Autodesk Inventor part; units mm, degrees
ref_plane "YZ Plane" through (0, 0, 0) normal (1, 0, 0) x (0, 1, 0)
ref_plane "XZ Plane" through (0, 0, 0) normal (0, 1, 0) x (-1, 0, 0)
ref_plane "XY Plane" through (0, 0, 0) normal (0, 0, 1) x (1, 0, 0)
sketch "Sketch2" plane through (0, 0, 0) normal (0, 1, 0) x (-1, 0, 0)
  circle A0 centre (0, 0) radius 22
  circle A1 centre (0, 0) radius 30
  dimension "d0" = 44
  dimension "d1" = 60
extrude "Extrusion1" add sketch "Sketch2" along normal blind 10
sketch "Sketch3" plane through (0, 10, 0) normal (0, 1, 0) x (1, 0, 0)
  circle A0 centre (0, 0) radius 30
  circle A1 centre (0, 0) radius 15
  dimension "d4" = 30
extrude "Extrusion2" add sketch "Sketch3" along normal blind 10
sketch "Sketch4" plane through (0, 20, 0) normal (0, 1, 0) x (1, 0, 0)
  circle A0 centre (0, 0) radius 25.1
  circle A1 centre (0, 0) radius 30
  dimension "d7" = 60
  dimension "d8" = 50.2
extrude "Extrusion3" add sketch "Sketch4" along normal blind 5
properties part number "smallbearingcup" material "Steel"
Here's how the part is built. I have some questions about the finished solid (model axes, mm). A direction names the side the tool comes from. Round coordinates to 2 decimals unless told otherwise and drop trailing zeros. Order: outer loops, then holes, each group sorted by start corner. A loop starts at its lowest first (then second) coordinate and runs counter-clockwise, first axis right, second up. Notation, with made-up numbers: M 39.25,76 L 59.25,76 A21 cw 59.25,113 Z; hole C 40,42.25 d6. An arc over 180 degrees is marked long. One line per question, with ' | ' between items.
1) I need wall thicknesses on line 1 (X direction, y = 17.25, z = 0); line 2 (X direction, y = 7.5, z = -0.5); line 3 (Z direction, x = 0, y = 22.65). Which ranges of each line are inside material? Lowest first, please.
Checked values:
line 1: x = -30 to -15, 15 to 30 | line 2: x = -30 to -21.99, 21.99 to 30 | line 3: z = -30 to -25.1, 25.1 to 30
2) Imagine slicing it at D-D, the plane y = 20.75. Write out the boundary of the cut face in (x, z).
Checked values:
outline: C 0,0 d60; hole C 0,0 d50.2
3) Imagine slicing it at B-B, the plane y = 11.5. Write out the boundary of the cut face in (x, z).
Checked values:
outline: C 0,0 d60; hole C 0,0 d30
4) On a 3-axis mill with a long thin cutter (end or side, diameter ignored), from which of +Z, -Z, +X, -X, +Y, -Y can I reach the whole of each face in a straight line? I mean faces 1 (the flat face through (14.4, 10, -5.2)), 2 (the flat face through (11, 20, 11)), 3 (the flat face through (-18, 25, 18)). Say none if no direction works.
Checked values:
face 1: -Y | face 2: +Y | face 3: +Z, -Z, +X, -X, +Y
5) I'm going to push flat-ended pins straight in: pin 1 Ø5 at (y, z) = (18.5, 16) entering from -X; pin 2 Ø1 at (y, z) = (18, -3) entering from -X; pin 3 Ø8 at (x, y) = (-9.5, 6.5) entering from +Z; pin 4 Ø25 at (x, z) = (-1, 0) entering from +Y. Where does each tip first touch, or does it pass through?
Checked values:
pin 1: stops at x = -26.79 | pin 2: stops at x = -29.9 | pin 3: stops at z = 29.49 | pin 4: passes through
6) We'd pull the mould along X, two halves only. Please class faces 4 (the flat face through (16, 0, 16)), 5 (the cylindrical face through (23.186, 22.465, -9.613)): released by +X, released by -X, zero draft, split by the parting line, or undercut.
Checked values:
face 4: zero draft | face 5: undercut
7) Imagine slicing it at A-A, the plane z = -12. Write out the boundary of the cut face in (x, y), plus the area to 3 significant figures.
Checked values:
outline: M -27.5,0 L -18.44,0 L -18.44,10 L -9,10 L -9,20 L -22.05,20 L -22.05,25 L -27.5,25 Z; M 9,10 L 18.44,10 L 18.44,0 L 27.5,0 L 27.5,25 L 22.05,25 L 22.05,20 L 9,20 Z | area: 606 mm²
